```python
from build123d import *

# Parameters (mm, degrees)
SKETCH1_W           = 45
SKETCH1_H           = 20.5
BOSS_EXTRUDE1_DEPTH = 1
SKETCH3_R           = 8.25
BOSS_EXTRUDE2_DEPTH = 12
BOSS_EXTRUDE3_DEPTH = 3.5
SKETCH6_W           = 39.311963292
SKETCH6_H           = 11.9190527
BOSS_EXTRUDE4_DEPTH = 2.5
SKETCH7_W           = 10
SKETCH7_H           = 3
BOSS_EXTRUDE5_DEPTH = 3
SKETCH8_W           = 0.5
SKETCH8_H           = 0.5
BOSS_EXTRUDE6_DEPTH = 4
SKETCH9_W           = 9
SKETCH9_H           = 3
CUT_EXTRUDE1_DEPTH  = 4
SKETCH10_W          = 0.5
SKETCH10_H          = 0.5
BOSS_EXTRUDE7_DEPTH = 7.5


with BuildPart() as part:
    # Sketch1 → Boss-Extrude1 (new body)
    with BuildSketch(Plane.XY):
        Rectangle(SKETCH1_W, SKETCH1_H)
    extrude(amount=BOSS_EXTRUDE1_DEPTH)

    # Sketch3 → Boss-Extrude2 (add)
    with BuildSketch(Plane(origin=(0, 0, 0), x_dir=(-1, 0, 0), z_dir=(0, 0, -1))):
        with Locations((12.25, 0)):
            Circle(SKETCH3_R)
    extrude(amount=BOSS_EXTRUDE2_DEPTH)

    # Sketch4 → Boss-Extrude3 (add)
    with BuildSketch(Plane(origin=(0, 0, 0), x_dir=(-1, 0, 0), z_dir=(0, 0, -1))):
        with BuildLine():
            Line((-7.639519339, 9.518507805), (2.360480661, 9.518507805))
            ThreePointArc((2.360480661, 9.518507805), (4.360480661, 7.518507805), (2.360480661, 5.518507805))
            Line((2.360480661, 5.518507805), (-7.639519339, 5.518507805))
            ThreePointArc((-7.639519339, 5.518507805), (-9.639519339, 7.518507805), (-7.639519339, 9.518507805))
        make_face()
    extrude(amount=BOSS_EXTRUDE3_DEPTH)

    # Sketch6 → Boss-Extrude4 (add)
    with BuildSketch(Plane.XY.offset(1)):
        Rectangle(SKETCH6_W, SKETCH6_H)
    extrude(amount=BOSS_EXTRUDE4_DEPTH)

    # Sketch7 → Boss-Extrude5 (add)
    with BuildSketch(Plane.XY.offset(1)):
        with Locations((0, -8.75)):
            Rectangle(SKETCH7_W, SKETCH7_H)
    extrude(amount=BOSS_EXTRUDE5_DEPTH)

    # Sketch8 → Boss-Extrude6 (add)
    with BuildSketch(Plane.XY.offset(4)):
        with Locations((-3.75, -8.75)):
            Rectangle(SKETCH8_W, SKETCH8_H)
        with Locations((-1.25, -8.75)):
            Rectangle(SKETCH8_W, SKETCH8_H)
        with Locations((1.25, -8.75)):
            Rectangle(SKETCH8_W, SKETCH8_H)
        with Locations((3.75, -8.75)):
            Rectangle(SKETCH8_W, SKETCH8_H)
    extrude(amount=BOSS_EXTRUDE6_DEPTH)

    # Sketch9 → Cut-Extrude1 (cut)
    with BuildSketch(Plane.XZ.offset(10.25)):
        with Locations((-0.5, 6.5)):
            Rectangle(SKETCH9_W, SKETCH9_H)
    extrude(amount=-CUT_EXTRUDE1_DEPTH, mode=Mode.SUBTRACT)

    # Sketch10 → Boss-Extrude7 (add)
    with BuildSketch(Plane.XZ.offset(9)):
        with Locations((-3.75, 4.75)):
            Rectangle(SKETCH10_W, SKETCH10_H)
        with Locations((-1.25, 4.75)):
            Rectangle(SKETCH10_W, SKETCH10_H)
        with Locations((1.25, 4.75)):
            Rectangle(SKETCH10_W, SKETCH10_H)
        with Locations((3.75, 4.75)):
            Rectangle(SKETCH10_W, SKETCH10_H)
    extrude(amount=BOSS_EXTRUDE7_DEPTH)


solid = part.part
```
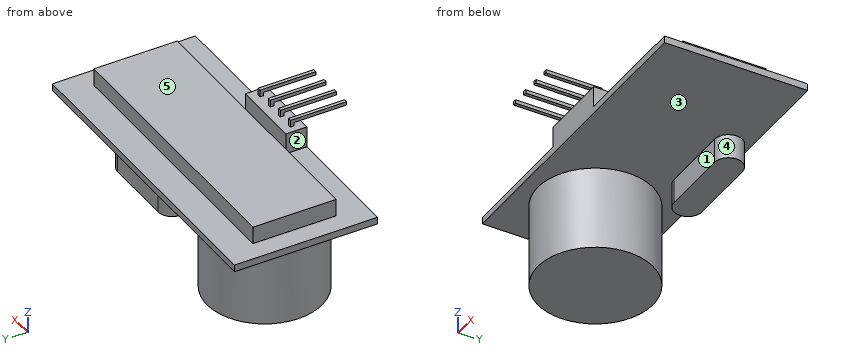
Model file for the job. Use its own axes, mm. Face numbers are marked on the shaded views. A direction names the side the tool comes from. Give positions to 0.01 mm unless a question says otherwise; leave off trailing zeros. Write each loop counter-clockwise with the first axis right and the second up, starting at its lowest first coordinate (ties: lowest second). Pieces come first, ordered by that corner, then holes. Notation, with made-up numbers: (35, 29) - (60, 29) arc R18 cw to (60, 48) - close; hole circle Ø10 at (-35.75, 40.25). An arc over 180 degrees is marked (long way). One line per question, with ' | ' between items. Start each with the question number.
(1) Slice it at A-A on z = 1.5. Write the cut outline in (x, y), plus the area to 3 significant figures.
(2) Pin check, flat tips, straight feed: P1, Ø9.5, axis at x = 1.5, y = 0.5, coming from the +Z side; P2, Ø3, axis at x = 2.5, z = -2.5, coming from the -Y side; P3, Ø4, axis at y = -5.5, z = -2.5, coming from the +X side; P4, Ø2, axis at x = 7, z = -6, coming from the +Y side. Stop position of each tip, or through.
(3) Slice it at C-C on y = 3. Write the cut outline in (x, z), plus the area to 3 significant figures.
(4) Slice it at B-B on x = -12.25. Write the cut outline in (y, z), plus the area to 3 significant figures.
(5) Wall check: line 1 along Y through (x, z) = (9, 0.5); line 2 along Z through (x, y) = (11, 0.25); line 3 along Z through (x, y) = (-1, 7). Give the ranges that are in metal, low to high. Write a range as from..to.
(6) 3-axis set-ups, long thin cutter, end or side, ignore diameter. For the marked faces 1, 2, 3, 4 and 5: which of +Z, -Z, +X, -X, +Y, -Y reach the whole face in a straight line?
(7) Slice it at D-D on z = -2. Write the cut outline in (x, y).
Results below:
1) outline: (-19.66, -5.96) - (19.66, -5.96) - (19.66, 5.96) - (-19.66, 5.96) - close; (-5, -10.25) - (5, -10.25) - (5, -7.25) - (-5, -7.25) - close | area: 499 mm^2
2) P1: z = 3.5 | P2: y = 5.52 | P3: x = -4.78 | P4: through
3) outline: (-22.5, 0) - (-19.94, 0) - (-19.94, -12) - (-4.56, -12) - (-4.56, 0) - (22.5, 0) - (22.5, 1) - (19.66, 1) - (19.66, 3.5) - (-19.66, 3.5) - (-19.66, 1) - (-22.5, 1) - close | area: 328 mm^2
4) outline: (-10.25, 0) - (-8.25, 0) - (-8.25, -12) - (8.25, -12) - (8.25, 0) - (10.25, 0) - (10.25, 1) - (5.96, 1) - (5.96, 3.5) - (-5.96, 3.5) - (-5.96, 1) - (-10.25, 1) - close | area: 248 mm^2
5) line 1: -10.25..10.25 | line 2: 0..3.5 | line 3: -3.5..1
6) face 1: -Z, +X, -Y | face 2: +Z, -X, -Y | face 3: -Z | face 4: -Z, +X | face 5: +Z, +X, -X, +Y
7) outline: circle Ø16.5 at (-12.25, 0); (-2.36, 5.52) - (7.64, 5.52) arc R2 ccw to (7.64, 9.52) - (-2.36, 9.52) arc R2 ccw to start
